Source: CAD feature listing. Evaluate the final solid. Frame: model axes, mm. A direction names the side the tool comes from. Round coordinates to 2 decimals unless told otherwise and drop trailing zeros. Loops run counter-clockwise (first coordinate to the right, second up) from the corner with the lowest first, then second, coordinate; pieces in that order, holes last. Notation, with made-up numbers: (67, 31.25) - (76, 31.25) arc R14 ccw to (76, 50.25) - close; hole circle Ø7 at (-21.75, 75.5). An arc over 180 degrees is marked (long way). Write item = value, one per line. Start each with the question number.
from build123d import *

# Parameters (mm, degrees)
SKETCH1_W           = 53.975
SKETCH1_H           = 53.975
BOSS_EXTRUDE1_DEPTH = 3.175
SKETCH2_W           = 3.175
SKETCH2_H           = 50.8
SKETCH2_W_2         = 50.8
SKETCH2_H_2         = 3.175
BOSS_EXTRUDE2_DEPTH = 25.4
CHAMFER1_SIZE       = 3.81
SKETCH3_R           = 3.175
CUT_EXTRUDE1_DEPTH  = 25.4


with BuildPart() as part:
    # Sketch1 → Boss-Extrude1 (new body)
    with BuildSketch(Plane(origin=(0, 0, 0), x_dir=(1, 0, 0), z_dir=(0, 1, 0))):
        with Locations((26.9875, 26.9875)):
            Rectangle(SKETCH1_W, SKETCH1_H)
    extrude(amount=BOSS_EXTRUDE1_DEPTH)

    # Sketch2 → Boss-Extrude2 (add)
    with BuildSketch(Plane(origin=(0, 3.175, 0), x_dir=(1, 0, 0), z_dir=(0, 1, 0))):
        with Locations((1.5875, 28.575)):
            Rectangle(SKETCH2_W, SKETCH2_H)
        with Locations((28.575, 1.5875)):
            Rectangle(SKETCH2_W_2, SKETCH2_H_2)
        with Locations((1.5875, 1.5875)):
            Rectangle(SKETCH2_W, SKETCH2_H_2)
    extrude(amount=BOSS_EXTRUDE2_DEPTH)

    # Chamfer1
    chamfer1_edges = [part.edges().sort_by_distance(p)[0] for p in [
        (0, 14.2875, 0),
    ]]
    chamfer(chamfer1_edges, length=CHAMFER1_SIZE)

    # Sketch3 → Cut-Extrude1 (cut)
    with BuildSketch(Plane(origin=(0, 3.175, 0), x_dir=(1, 0, 0), z_dir=(0, 1, 0))):
        with Locations(Location((22.352, 47.625, 0), (0, 0, 270))):
            Circle(SKETCH3_R)
        with Locations(Location((47.625, 22.352, 0), (0, 0, 270))):
            Circle(SKETCH3_R)
    extrude(amount=-CUT_EXTRUDE1_DEPTH, mode=Mode.SUBTRACT)


solid = part.part
(1) Pin query (flat end, axial travel): P1, Ø12, axis at y = 24.5, z = -14, coming from the +X side (3 decimals); P2, Ø7.5, axis at x = 38, y = 14.5, coming from the -Z side (3 decimals); P3, Ø1, axis at x = 37, z = -31, coming from the +Y side (3 decimals). Return the tip coordinate at first contact, or that it passes through.
(2) Cut plane A-A (y = 9). Output: boundary loops of the cut face in (x, z) (3 decimals), and give its area (3 significant figures).
(3) Cut plane D-D (x = 12.5). Output: boundary loops of the cut face in (y, z) (3 decimals), and give its area (3 significant figures).
(4) Material intervals for line 1 along Z through (x, y) = (18, 8.5) (3 decimals); line 2 along Y through (x, z) = (35.5, -5.5) (3 decimals), sorted ascending. Write a range as from..to.
(5) Cut plane C-C (y = 2.5). Output: boundary loops of the cut face in (x, z) (3 decimals).
(6) Cut plane B-B (z = -47). Output: boundary loops of the cut face in (x, y) (3 decimals).
(7) Mould query, pull axis Z, two halves, no side actions, for faces 1 (the face through (44.8, 1.6, -20.9)), 2 (the face through (15, 3, -53.975)), 3 (the face through (0, 14, -29)). Classes: +Z half, -Z half, draft (parallel to the pull), parting line (faces both ways), or undercut.
(8) Access query for faces 4 (the face through (28, 16, -3.175)), 5 (the face through (3, 28.575, -15)). Directions: +Z, -Z, +X, -X, +Y, -Y. A direction counts if a zero-diameter tool reaches every point of the face in a straight line with its end or side. Return the directions, or none.
Solution:
q1.P1 = 3.175
q1.P2 = -3.175
q1.P3 = 3.175
q2.outline = (0, -53.975) - (3.175, -53.975) - (3.175, -3.175) - (53.975, -3.175) - (53.975, 0) - (3.81, 0) - (0, -3.81) - close
q2.area = 325 mm^2
q3.outline = (0, -53.975) - (3.175, -53.975) - (3.175, -3.175) - (28.575, -3.175) - (28.575, 0) - (0, 0) - close
q3.area = 252 mm^2
q4.line_1 = -3.175..0
q4.line_2 = 0..3.175
q5.outline = (0, -53.975) - (53.975, -53.975) - (53.975, 0) - (3.81, 0) - (0, -3.81) - close; hole circle Ø6.35 at (22.352, -47.625); hole circle Ø6.35 at (47.625, -22.352)
q6.outline = (0, 0) - (19.239, 0) - (19.239, 3.175) - (3.175, 3.175) - (3.175, 28.575) - (0, 28.575) - close; (25.465, 0) - (53.975, 0) - (53.975, 3.175) - (25.465, 3.175) - close
q7.face_1 = undercut
q7.face_2 = -Z half
q7.face_3 = draft
q8.face_4 = -Z, +X, +Y
q8.face_5 = +Z, -Z, +X, -X, +Y
